Here's how the part is built. I have some questions about the finished solid (model axes, mm). A direction names the side the tool comes from. Coordinates: 2 decimals unless noted, no trailing zeros. Loops run counter-clockwise (first coordinate to the right, second up) from the corner with the lowest first, then second, coordinate; pieces in that order, holes last. Notation, with made-up numbers: (17, -3.75) -> (43, -3.75) arc R37 ccw to (43, 35.25) -> close; hole circle Ø9 at (30.25, 80.25). An arc over 180 degrees is marked (long way). Answer as a JSON object with one key per item and string values. Group by question number.
Q1. I want a section at A-A on y = 0. Write out the boundary of the cut face in (x, z), then the cut area to 3 significant figures.
Q2. I want a section at D-D on z = 7.75. Write out the boundary of the cut face in (x, y).
Q3. I'm going to push flat-ended pins straight in: pin 1 (2 mm diameter, centred on y = -0.5, z = 6, fed in from -X); pin 2 (1 mm diameter, centred on y = 1.5, z = 2.5, fed in from -X); pin 3 (1.5 mm diameter, centred on y = 2, z = 7.5, fed in from -X). Where does each tip first touch, or does it pass through?
Q4. I want a section at C-C on z = 5.75. Write out the boundary of the cut face in (x, y).
Q5. I need wall thicknesses on line 1 (Z direction, x = 0.7, y = 2.6); line 2 (X direction, y = 0.05, z = 4); line 3 (Z direction, x = -1.8, y = -1.4). Which ranges of each line are inside material? Lowest first, please.
Q6. On a 3-axis mill with a long thin cutter (end or side, diameter ignored), from which of +Z, -Z, +X, -X, +Y, -Y can I reach the whole of each face in a straight line? I mean faces 1 (the cylindrical face through (-3, 0.1, 0.2)), 2 (the flat face through (-2, 2, 0.5)). Say none if no direction works.
```python
from build123d import *

# Parameters (mm, degrees)
CYLINDER001_R     = 3
CYLINDER001_DEPTH = 0.5
CYLINDER_R        = 2.5
CYLINDER_DEPTH    = 6


with BuildPart() as sphere:
    # Sphere → Sphere (revolve)
    with BuildSketch(Plane(origin=(0, 0, 6), x_dir=(1, 0, 0), z_dir=(0, -1, 0))):
        with BuildLine():
            ThreePointArc((0, -2.5), (2.5, 0), (0, 2.5))
            Line((0, 2.5), (0, -2.5))
        make_face()
    revolve(axis=Axis((0, 0, 6), (0, 0, 1)))


with BuildPart() as cylinder001:
    # Cylinder001 → Cylinder001 (new body)
    with BuildSketch(Plane.XY):
        Circle(CYLINDER001_R)
    extrude(amount=CYLINDER001_DEPTH)


with BuildPart() as led_5mm:
    # Cylinder → Cylinder (new body)
    with BuildSketch(Plane.XY):
        Circle(CYLINDER_R)
    extrude(amount=CYLINDER_DEPTH)

    # Fusion: union Sphere, Cylinder001
    add(sphere.part)
    add(cylinder001.part)


solid = led_5mm.part
```
Result set:
{
 "1": {"outline": "(-3, 0) -> (3, 0) -> (3, 0.5) -> (2.5, 0.5) -> (2.5, 6) arc R2.5 ccw to (-2.5, 6) -> (-2.5, 0.5) -> (-3, 0.5) -> close", "area": "40.3 mm²"},
 "2": {"outline": "circle Ø3.57 at (0, 0)"},
 "3": {"pin 1": "stops at x = -2.5", "pin 2": "stops at x = -2.29", "pin 3": "stops at x = -1.79"},
 "4": {"outline": "circle Ø5 at (0, 0)"},
 "5": {"line 1": "z = 0 to 0.5", "line 2": "x = -2.5 to 2.5", "line 3": "z = 0 to 7.02"},
 "6": {"face 1": "+Z, -Z", "face 2": "+Z"}
}
